Autodesk Inventor part; units mm, degrees
ref_plane "YZ Plane" through (0, 0, 0) normal (1, 0, 0) x (0, 1, 0)
ref_plane "XZ Plane" through (0, 0, 0) normal (0, 1, 0) x (-1, 0, 0)
ref_plane "XY Plane" through (0, 0, 0) normal (0, 0, 1) x (1, 0, 0)
ref_plane "Work Plane1" through (-41.89, 79.898, 0.7952) normal (0, 0, 1) x (1, 0, 0)
sketch "Sketch1" plane through (-41.89, 79.898, 0.7952) normal (0, 0, 1) x (1, 0, 0)
  circle A0 centre (41.89, -79.898) radius 1.45
  circle A1 centre (8.87, -27.828) radius 1.45
  circle A2 centre (57.13, -29.098) radius 1.45
  arc A3 (66, -80.398) -> (68, -78.398) centre (66, -78.398) ccw
  line L0 (66, 0.102) -> (0, 0.102)
  line L1 (-2, -1.898) -> (-2, -24.398)
  line L2 (-2, 0.102) -> (68, 0.102)
  line L3 (68, 0.102) -> (68, -82.398)
  line L4 (68, -82.398) -> (-2, -82.398)
  line L5 (-2, -82.398) -> (-2, 0.102)
  line L6 (-2, 3.102) -> (-5, 3.102)
  line L7 (68, -85.398) -> (71, -85.398)
  line L8 (-5, 3.102) -> (71, 3.102)
  line L9 (71, 3.102) -> (71, -85.398)
  line L10 (71, -85.398) -> (-5, -85.398)
  line L11 (-5, -85.398) -> (-5, 3.102)
  point P0 (44.5, -82.398)
  point P1 (-2, 3.102)
  point P2 (-2, -24.398)
  point P3 (-2, -1.898)
  point P4 (66, 0.102)
  dimension "d0" = 2.9
  dimension "d1" = 2.9
  dimension "d2" = 2.9
extrude "Extrusion1" add sketch "Sketch1" against normal blind 5 contours L2 L3 L4 L5 L1 L0 | L8 L9 L7 L10 L11 L6
sketch "Sketch2" plane through (-41.89, 79.898, 0.7952) normal (0, 0, 1) x (1, 0, 0)
  circle A0 centre (8.87, -27.828) radius 1.45
  circle A1 centre (8.87, -27.828) radius 3
  circle A2 centre (57.13, -29.098) radius 1.45
  circle A3 centre (57.13, -29.098) radius 3
  circle A4 centre (41.89, -79.898) radius 3
  circle A5 centre (41.89, -79.898) radius 1.45
  dimension "d9" = 6
  dimension "d10" = 6
  dimension "d11" = 6
extrude "Extrusion2" add sketch "Sketch2" along normal blind 3
sketch "Sketch3" plane through (-41.89, 79.898, 0.7952) normal (0, 0, 1) x (1, 0, 0)
  line L0 (71, -85.398) -> (-5, -85.398)
  circle A0 centre (18, -27.898) radius 1.45
  circle A1 centre (48, -27.898) radius 1.45
  circle A2 centre (18, -57.898) radius 1.45
  circle A3 centre (48, -57.898) radius 1.45
  point P0 (41.89, -79.898)
  dimension "d19" = 2.9
  dimension "d20" = 2.9
  dimension "d21" = 2.9
  dimension "d22" = 2.9
extrude "Extrusion3" cut sketch "Sketch3" against normal up to surface (5 mm away)
sketch "Sketch4" plane through (-41.89, 79.898, 0.7952) normal (0, 0, 1) x (1, 0, 0)
  circle A0 centre (18, -57.898) radius 1.45
  circle A1 centre (18, -57.898) radius 3
  circle A2 centre (18, -57.898) radius 1.45
  circle A3 centre (48, -57.898) radius 1.45
  circle A4 centre (48, -57.898) radius 1.45
  circle A5 centre (48, -57.898) radius 3
  circle A6 centre (48, -27.898) radius 1.45
  circle A7 centre (48, -27.898) radius 1.45
  circle A8 centre (48, -27.898) radius 3
  circle A9 centre (18, -27.898) radius 1.45
  circle A10 centre (18, -27.898) radius 1.45
  circle A11 centre (18, -27.898) radius 3
  point P0 (41.89, -79.898)
  dimension "d25" = 6
  dimension "d26" = 6
  dimension "d27" = 6
  dimension "d28" = 6
extrude "Extrusion4" cut sketch "Sketch4" against normal blind 2
extrude "Extrusion5" add sketch "Sketch1" along normal blind 4.58 contours L8 L9 L7 L10 L11 L6
properties part number "nucleo_din_connector"
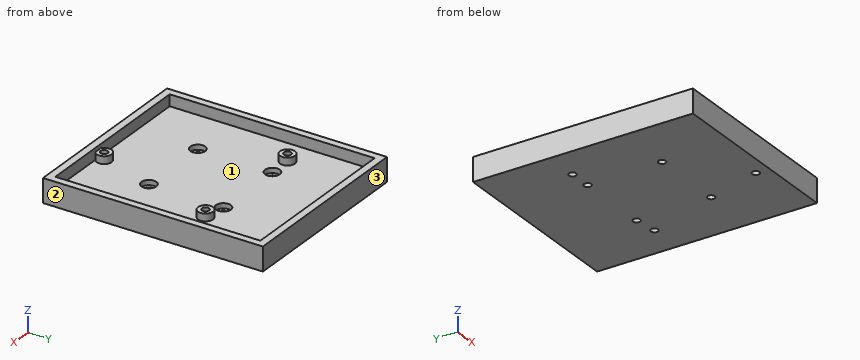
Here's how the part is built. I have some questions about the finished solid (model axes, mm). Face numbers are marked on the shaded views. Coordinates: 2 decimals unless noted, no trailing zeros. Loops run counter-clockwise (first coordinate to the right, second up) from the corner with the lowest first, then second, coordinate; pieces in that order, holes last.
1. If we mould it in two halves opening along X, with no side actions, what happens to the marked faces 1, 2 and 3? For each: pulls with the +X half, pulls with the -X half, needs draft (parallel to the pull), parting line crosses it, or undercut.
2. I need wall thicknesses on L1, parallel to Y at x = 6.11, z = -2.4; L2, parallel to Y at x = 6.11, z = -0.1; L3, parallel to X at y = 16, z = 2.75. Which ranges of each line are inside material? Lowest first, please.
3. Imagine slicing it at A-A, the plane x = 15.24. Please give me the cut outline in (y, z).
4. Imagine slicing it at D-D, the plane z = -0.25. Please give me the cut outline in (x, y).
5. For P1, Ø2.5, axis at x = 0, y = 0, coming from the +Z side; P2, Ø1, axis at x = -13, y = 51.5, coming from the +Z side; P3, Ø5, axis at x = -32, y = 52, coming from the +Z side; P4, Ø3, axis at x = 6, y = 23, coming from the +Z side, each with a flat end and sliding along its axis, tell me the tip position at first contact or that it passes through.
6. Imagine slicing it at B-B, the plane x = -23.89. Please give me the cut outline in (y, z).
7. Imagine slicing it at C-C, the plane y = 22. Please give me the cut outline in (x, z), and give its area (3 significant figures).
Taken from the geometry:
1. face 1: undercut
1. face 2: pulls with the +X half
1. face 3: needs draft
2. L1: y = -5.5 to 20.55, 23.45 to 50.55, 53.45 to 83
2. L2: y = -5.5 to 19, 25 to 49, 55 to 83
2. L3: x = -46.89 to -43.89, 26.11 to 29.11
3. outline: (-5.5, -4.2) - (49.35, -4.2) - (49.35, 3.8) - (47.8, 3.8) - (47.8, 0.8) - (-2.5, 0.8) - (-2.5, 5.38) - (-5.5, 5.38) - close; (52.25, -4.2) - (83, -4.2) - (83, 5.38) - (80, 5.38) - (80, 0.8) - (53.8, 0.8) - (53.8, 3.8) - (52.25, 3.8) - close
4. outline: (-46.89, -5.5) - (29.11, -5.5) - (29.11, 83) - (-46.89, 83) - close; hole circle Ø2.9 at (-33.02, 52.07); hole circle Ø6 at (-23.89, 22); hole circle Ø6 at (-23.89, 52); hole circle Ø2.9 at (0, 0); hole circle Ø6 at (6.11, 22); hole circle Ø6 at (6.11, 52); hole circle Ø2.9 at (15.24, 50.8)
5. P1: passes through
5. P2: stops at z = 0.8
5. P3: stops at z = 3.8
5. P4: stops at z = -1.2
6. outline: (-5.5, -4.2) - (20.55, -4.2) - (20.55, -1.2) - (19, -1.2) - (19, 0.8) - (-2.5, 0.8) - (-2.5, 5.38) - (-5.5, 5.38) - close; (23.45, -4.2) - (50.55, -4.2) - (50.55, -1.2) - (49, -1.2) - (49, 0.8) - (25, 0.8) - (25, -1.2) - (23.45, -1.2) - close; (53.45, -4.2) - (83, -4.2) - (83, 5.38) - (80, 5.38) - (80, 0.8) - (55, 0.8) - (55, -1.2) - (53.45, -1.2) - close
7. outline: (-46.89, -4.2) - (-25.34, -4.2) - (-25.34, -1.2) - (-26.89, -1.2) - (-26.89, 0.8) - (-43.89, 0.8) - (-43.89, 5.38) - (-46.89, 5.38) - close; (-22.44, -4.2) - (4.66, -4.2) - (4.66, -1.2) - (3.11, -1.2) - (3.11, 0.8) - (-20.89, 0.8) - (-20.89, -1.2) - (-22.44, -1.2) - close; (7.56, -4.2) - (29.11, -4.2) - (29.11, 5.38) - (26.11, 5.38) - (26.11, 0.8) - (9.11, 0.8) - (9.11, -1.2) - (7.56, -1.2) - close
7. area: 366 mm2
